Autodesk Inventor part; units mm, degrees
sketch "Sketch1" plane through (0, 0, 0) normal (0, 0, 1) x (1, 0, 0)
  line L0 (-4.55, 7.5) -> (4.55, 7.5)
  line L1 (4.55, 7.5) -> (4.55, -7.5)
  line L2 (4.55, -7.5) -> (-4.55, -7.5)
  line L3 (-4.55, -7.5) -> (-4.55, 7.5)
  line L4 (-4.55, 7.5) -> (4.55, -7.5) construction
  line L5 (4.55, 7.5) -> (-4.55, -7.5) construction
  line L6 (-2.05, -2.05) -> (2.05, -2.05)
  line L7 (2.05, -2.05) -> (2.05, 2.05)
  line L8 (2.05, 2.05) -> (-2.05, 2.05)
  line L9 (-2.05, 2.05) -> (-2.05, -2.05)
  line L10 (-2.05, -2.05) -> (2.05, 2.05) construction
  line L11 (2.05, -2.05) -> (-2.05, 2.05) construction
  line L12 (-4.55, 7.5) -> (-16.55, 7.5)
  line L13 (-16.55, 7.5) -> (-16.55, 6)
  line L14 (-16.55, 6) -> (-4.55, 6)
  line L15 (-4.55, 6) -> (-4.55, 7.5)
  line L16 (-4.55, -7.5) -> (-16.55, -7.5)
  line L17 (-16.55, -7.5) -> (-16.55, -6)
  line L18 (-16.55, -6) -> (-4.55, -6)
  line L19 (-4.55, -6) -> (-4.55, -7.5)
  line L20 (4.55, 7.5) -> (16.55, 7.5)
  line L21 (16.55, 7.5) -> (16.55, 6)
  line L22 (16.55, 6) -> (4.55, 6)
  line L23 (4.55, 6) -> (4.55, 7.5)
  line L24 (4.55, -7.5) -> (16.55, -7.5)
  line L25 (16.55, -7.5) -> (16.55, -6)
  line L26 (16.55, -6) -> (4.55, -6)
  line L27 (4.55, -6) -> (4.55, -7.5)
  point P0 (0, 0)
  point P1 (-4.55, 6)
  point P2 (-4.55, -6)
  point P3 (4.55, 6)
  dimension "d0" = 15
  dimension "d1" = 9.1
  dimension "d2" = 4.1
  dimension "d3" = 4.1
  dimension "d4" = 12
  dimension "d5" = 1.5
  dimension "d8" = 1.5
  dimension "d9" = 12
  dimension "d10" = 12
  dimension "d11" = 1.5
  dimension "d12" = 12
extrude "Extrusion1" add sketch "Sketch1" along normal blind 12
sketch "Sketch3" plane through (4.55, -6, 0) normal (1, 0, 0) x (0, 0, -1)
  line L0 (-6.4, 3.1) -> (-5.6, 3.1)
  line L1 (-5.6, 3.1) -> (-5.6, 0)
  line L2 (-5.6, 0) -> (-6.4, 0)
  line L3 (-6.4, 0) -> (-6.4, 3.1)
  line L4 (0, 12) -> (-12, 12)
  line L5 (0, 0) -> (0, 12)
  line L6 (0, 0) -> (-12, 0)
  point P0 (0, 6)
  dimension "d24" = 3.1
  dimension "d25" = 0.8
  dimension "d30" = 0
  dimension "d39" = 12
  dimension "d40" = 5.6
extrude "Extrusion3" cut sketch "Sketch3" against normal through all
sketch "Sketch5" plane through (0, 0, 0) normal (0, 0, -1) x (-1, 0, 0)
  line L0 (-2.05, 5.05) -> (2.05, 5.05)
  line L1 (2.05, 5.05) -> (2.05, 3.55)
  line L2 (2.05, 3.55) -> (-2.05, 3.55)
  line L3 (-2.05, 3.55) -> (-2.05, 5.05)
  line L4 (-2.05, -3.55) -> (2.05, -3.55)
  line L5 (2.05, -3.55) -> (2.05, -5.05)
  line L6 (2.05, -5.05) -> (-2.05, -5.05)
  line L7 (-2.05, -5.05) -> (-2.05, -3.55)
  line L8 (2.05, 2.05) -> (-2.05, 2.05)
  line L9 (2.05, -2.05) -> (2.05, 2.05)
  line L10 (-2.05, -2.05) -> (2.05, -2.05)
  point P0 (0, 0)
  dimension "d31" = 4.1
  dimension "d32" = 4.1
  dimension "d33" = 1.5
  dimension "d34" = 1.5
  dimension "d35" = 1.5
  dimension "d36" = 1.5
extrude "Extrusion4" cut sketch "Sketch5" against normal through all
fillet "Fillet2" radius 2 8 edges at (-16.55, 6.75, 0) (-16.55, 6.75, 12) (-16.55, -6.75, 0) (-16.55, -6.75, 12) (16.55, 6.75, 12) (16.55, -6.75, 12) (16.55, 6.75, 0) (16.55, -6.75, 0)
equation "\"d40\" = -0.5 * d25 + 0.5 * d39"
equation "\"d31\" = d32"
properties part number "wing_clamp_interface"
The listing builds one solid part. Answer for the finished solid, in the listing's coordinates (mm). A direction names the side the tool comes from. Coordinates: 2 decimals unless noted, no trailing zeros. Loops run counter-clockwise (first coordinate to the right, second up) from the corner with the lowest first, then second, coordinate; pieces in that order, holes last. Notation, with made-up numbers: (53.5, 36.25) -> (111.5, 36.25) arc R24 ccw to (111.5, 74.25) -> close; hole circle Ø4 at (23, 83.5). An arc over 180 degrees is marked (long way). Answer in a Markdown table with one row per item. Add a question column.
1. The part is cut by section A-A, the plane y = 0. Write down the section's boundary in (x, z), then the cut area to 3 significant figures.
2. The part is cut by section B-B, the plane x = -8. Write down the section's boundary in (y, z).
3. The part is cut by section C-C, the plane z = 9.5. Write down the section's boundary in (x, y), then the cut area to 3 significant figures.
4. For faces 4 (the flat face through (0.1, -5.2, 6.4)), 5 (the flat face through (0, 5.05, 6)), 6 (the flat face through (-11, 6, 6)), 7 (the flat face through (11, 6, 6)), 8 (the flat face through (-16.55, 7, 6)), determine the directions among +Z, -Z, +X, -X, +Y, -Y from which every point of the face is accessible in a straight line to the end or side of a thin tool.
5. The part is cut by section D-D, the plane z = 1.5. Write down the section's boundary in (x, y).
6. Determine the mould class of faces 1 (the cylindrical face through (-15.98, 6.74, 0.6)), 2 (the flat face through (4.55, 0, 6)), 3 (the flat face through (0, 3.55, 6)) for opening direction X: +X half, -X half, draft (parallel to the pull), parting line (faces both ways), or undercut.
7. Flat-ended cylindrical pins translate along their axes: P1, Ø6, axis at y = 1.5, z = 5, coming from the +X side; P2, Ø6, axis at y = -1.5, z = 8, coming from the -X side. Find the tip coordinate at first contact, or state that the pin passes through.
8. Consider line 1 (Y direction, x = 2, z = 11.25); line 2 (Y direction, x = -7, z = 11); line 3 (X direction, y = 0.25, z = 4.75). Determine where each line is inside the solid, lowest interval first. Write a range as [from, to].
Answer below:
| question | item | result |
|---|---|---|
| 1 | outline | (-4.55, 0) -> (-2.05, 0) -> (-2.05, 12) -> (-4.55, 12) -> close; (2.05, 0) -> (4.55, 0) -> (4.55, 12) -> (2.05, 12) -> close |
| 1 | area | 60.0 mm2 |
| 2 | outline | (-7.5, 0) -> (-6, 0) -> (-6, 12) -> (-7.5, 12) -> close; (6, 0) -> (7.5, 0) -> (7.5, 12) -> (6, 12) -> close |
| 3 | outline | (-16.55, -7.5) -> (16.55, -7.5) -> (16.55, -6) -> (4.55, -6) -> (4.55, 6) -> (16.55, 6) -> (16.55, 7.5) -> (-16.55, 7.5) -> (-16.55, 6) -> (-4.55, 6) -> (-4.55, -6) -> (-16.55, -6) -> close; hole (-2.05, -5.05) -> (2.05, -5.05) -> (2.05, -3.55) -> (-2.05, -3.55) -> close; hole (-2.05, -2.05) -> (2.05, -2.05) -> (2.05, 2.05) -> (-2.05, 2.05) -> close; hole (-2.05, 3.55) -> (2.05, 3.55) -> (2.05, 5.05) -> (-2.05, 5.05) -> close |
| 3 | area | 179 mm2 |
| 4 | face 4 | +X, -X |
| 4 | face 5 | +Z, -Z |
| 4 | face 6 | +Z, -Z, -X |
| 4 | face 7 | +Z, -Z, +X |
| 4 | face 8 | +Z, -Z, -X, +Y, -Y |
| 5 | outline | (-16.49, -7.5) -> (16.49, -7.5) -> (16.49, -6) -> (4.55, -6) -> (4.55, 6) -> (16.49, 6) -> (16.49, 7.5) -> (-16.49, 7.5) -> (-16.49, 6) -> (-4.55, 6) -> (-4.55, -6) -> (-16.49, -6) -> close; hole (-2.05, -5.05) -> (2.05, -5.05) -> (2.05, -3.55) -> (-2.05, -3.55) -> close; hole (-2.05, -2.05) -> (2.05, -2.05) -> (2.05, 2.05) -> (-2.05, 2.05) -> close; hole (-2.05, 3.55) -> (2.05, 3.55) -> (2.05, 5.05) -> (-2.05, 5.05) -> close |
| 6 | face 1 | -X half |
| 6 | face 2 | +X half |
| 6 | face 3 | undercut |
| 7 | P1 | x = 4.55 |
| 7 | P2 | x = -4.55 |
| 8 | line 1 | [-7.5, -5.05], [-3.55, -2.05], [2.05, 3.55], [5.05, 7.5] |
| 8 | line 2 | [-7.5, -6], [6, 7.5] |
| 8 | line 3 | [-4.55, -2.05], [2.05, 4.55] |
